Could you check a few things on this drawing? It's one solid part, dimensions in mm from its lowest x, y, z. A direction names the side the tool comes from. Coordinates: 2 decimals unless noted, no trailing zeros. Write each loop counter-clockwise with the first axis right and the second up, starting at its lowest first coordinate (ties: lowest second). Pieces come first, ordered by that corner, then holes. Notation, with made-up numbers: M -23.5,15 L -18.5,15 A13 cw -18.5,35 Z; hole C -9,87 d9. An arc over 180 degrees is marked long. Use a Markdown table: item, result.
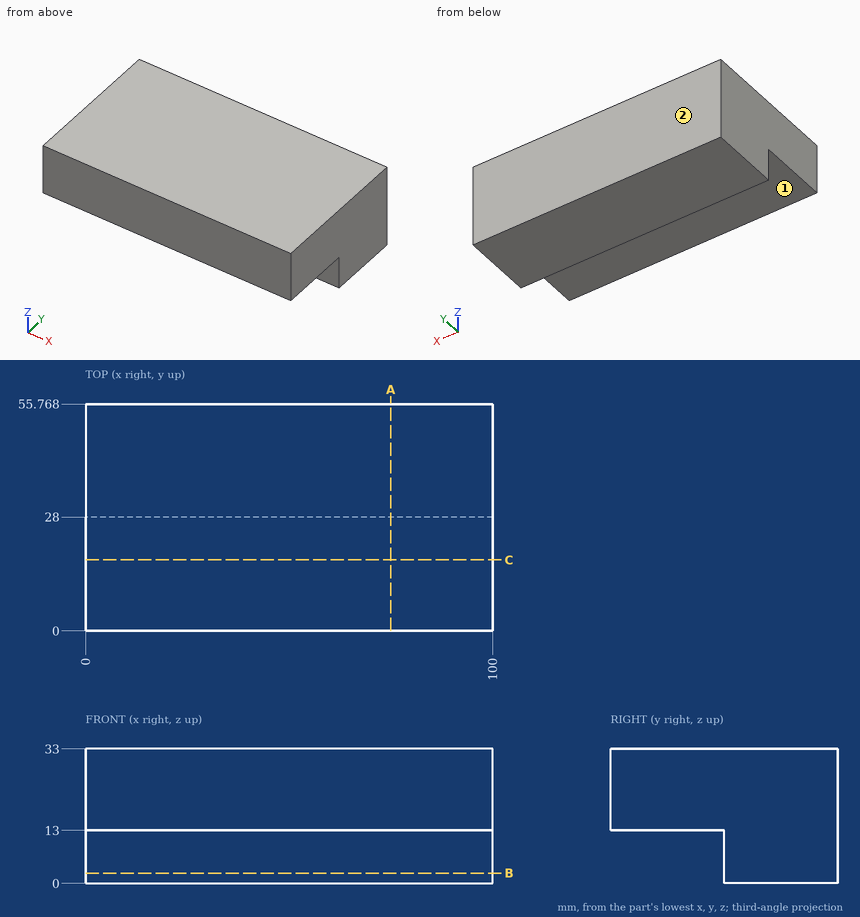
1. Will these pins go through, and if not, where does the flat tip stop? pin 1 Ø5 at (x, y) = (63.5, 11) entering from -Z; pin 2 Ø12 at (x, z) = (78, 6.5) entering from -Y.
Answers follow:
| item | result |
|---|---|
| pin 1 | stops at z = 13 |
| pin 2 | stops at y = 28 |
2. Suppose I cut it at C-C on y = 17.5. Write out the boundary of the cut face in (x, z).
Answers follow:
| item | result |
|---|---|
| outline | M 0,13 L 100,13 L 100,33 L 0,33 Z |
3. Which directions (+Z, -Z, +X, -X, +Y, -Y) give clear straight access to the entire face, cutting with the end or side of a thin tool? Please do the marked faces 1 and 2.
Answers follow:
| item | result |
|---|---|
| face 1 | -Z, +X, -X, -Y |
| face 2 | +Z, -Z, +X, -X, +Y |
4. I need wall thicknesses on probe 1 along Z at (x, y) = (83, 6.5); probe 2 along Y at (x, z) = (61, 9). Which ranges of each line are inside material? Lowest first, please.
Answers follow:
| item | result |
|---|---|
| probe 1 | z = 13 to 33 |
| probe 2 | y = 28 to 55.77 |
5. Suppose I cut it at A-A on x = 75. Write out the boundary of the cut face in (y, z).
Answers follow:
| item | result |
|---|---|
| outline | M 0,13 L 28,13 L 28,0 L 55.77,0 L 55.77,33 L 0,33 Z |
6. Suppose I cut it at B-B on z = 2.5. Write out the boundary of the cut face in (x, y).
Answers follow:
| item | result |
|---|---|
| outline | M 0,28 L 100,28 L 100,55.77 L 0,55.77 Z |
